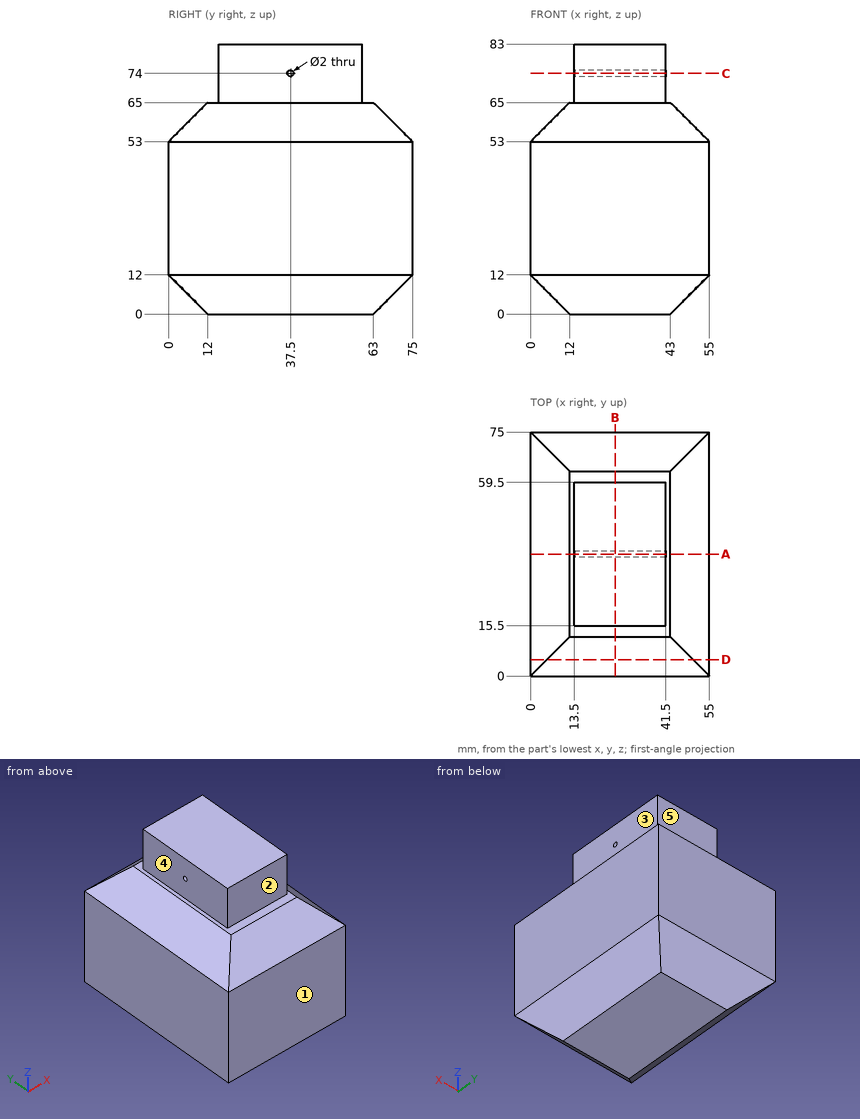
Can you work these out from the drawing? Everything is in mm from the part's minimum corner. A direction names the side the tool comes from. Give positions to 0.01 mm unless a question says otherwise; leave off trailing zeros. Loops run counter-clockwise (first coordinate to the right, second up) from the corner with the lowest first, then second, coordinate; pieces in that order, holes last. Notation, with made-up numbers: (10, 43) -> (37, 43) arc R24 ccw to (37, 82) -> close; hole circle Ø3 at (21.25, 27.5). An arc over 180 degrees is marked (long way). Return JSON: item names as keys, results as strings.
Q1. I need wall thicknesses on probe 1 along Y at (x, z) = (25.25, 74); probe 2 along Z at (x, y) = (35.75, 37.5); probe 3 along X at (y, z) = (19.5, 72). Which ranges of each line are inside material? Lowest first, please.
Checks:
{"probe 1": "y = 15.5 to 36.5, 38.5 to 59.5", "probe 2": "z = 0 to 73, 75 to 83", "probe 3": "x = 13.5 to 41.5"}
Q2. I want a section at B-B, the plane x = 26. List the corners of the cut face in (y, z) for me, then the cut area to 3 significant figures.
Checks:
{"outline": "(0, 12) -> (12, 0) -> (63, 0) -> (75, 12) -> (75, 53) -> (63, 65) -> (59.5, 65) -> (59.5, 83) -> (15.5, 83) -> (15.5, 65) -> (12, 65) -> (0, 53) -> close; hole circle Ø2 at (37.5, 74)", "area": "5,380 mm2"}
Q3. I want a section at A-A, the plane y = 37.5. List the corners of the cut face in (x, z) for me.
Checks:
{"outline": "(0, 12) -> (12, 0) -> (43, 0) -> (55, 12) -> (55, 53) -> (43, 65) -> (41.5, 65) -> (41.5, 73) -> (13.5, 73) -> (13.5, 65) -> (12, 65) -> (0, 53) -> close; (13.5, 75) -> (41.5, 75) -> (41.5, 83) -> (13.5, 83) -> close"}
Q4. I want a section at D-D, the plane y = 5. List the corners of the cut face in (x, z) for me.
Checks:
{"outline": "(0, 12) -> (5, 7) -> (50, 7) -> (55, 12) -> (55, 53) -> (50, 58) -> (5, 58) -> (0, 53) -> close"}
Q5. For pin 1 Ø9 at (y, z) = (36.5, 75.5) entering from +X; pin 2 Ø2 at (x, y) = (7.5, 30.5) entering from +Z; pin 3 Ø8 at (x, z) = (19.5, 73) entering from -Y, each with a flat end and sliding along its axis, tell me the tip position at first contact or that it passes through.
Checks:
{"pin 1": "stops at x = 41.5", "pin 2": "stops at z = 61.5", "pin 3": "stops at y = 15.5"}
Q6. I want a section at C-C, the plane z = 74. List the corners of the cut face in (x, y) for me, then the cut area to 3 significant figures.
Checks:
{"outline": "(13.5, 15.5) -> (41.5, 15.5) -> (41.5, 36.5) -> (13.5, 36.5) -> close; (13.5, 38.5) -> (41.5, 38.5) -> (41.5, 59.5) -> (13.5, 59.5) -> close", "area": "1,180 mm2"}
Q7. On a 3-axis mill with a long thin cutter (end or side, diameter ignored), from which of +Z, -Z, +X, -X, +Y, -Y can I reach the whole of each face in a straight line? I mean the marked faces 1, 2, 3, 4 and 5. Say none if no direction works.
Checks:
{"face 1": "+Z, -Z, +X, -X, -Y", "face 2": "+Z, +X, -X, -Y", "face 3": "+Z, +X, +Y, -Y", "face 4": "+Z, -X, +Y, -Y", "face 5": "+Z, +X, -X, +Y"}
